Read the model definition and answer for the solid it produces. Units are mm, in the model's axes. A direction names the side the tool comes from. Round coordinates to 2 decimals unless told otherwise and drop trailing zeros. Write each loop counter-clockwise with the first axis right and the second up, starting at its lowest first coordinate (ties: lowest second). Pieces come first, ordered by that corner, then holes.
from build123d import *
from build123d.topology import SkipClean

# Parameters (mm, degrees)
SALIENTE_EXTRUIR1_DEPTH    = 2.4
CORTAR_EXTRUIR1_DEPTH      = 36.210225787
CORTAR_EXTRUIR1_DEPTH_BACK = 36.210225787
CROQUIS2_R                 = 1.5
CROQUIS3_R                 = 1.5
SALIENTE_EXTRUIR2_DEPTH    = 7.5
CORTAR_EXTRUIR2_DEPTH      = 3.1
REDONDEO1_R                = 2
REDONDEO2_R                = 1


with BuildPart() as part:
    # Croquis1 → Saliente-Extruir1 (new, symmetric)
    with BuildSketch(Plane(origin=(0, 0, 0), x_dir=(0, 0, -1), z_dir=(1, 0, 0))):
        with BuildLine():
            Line((-34, 3), (34, 3))
            ThreePointArc((34, 3), (34.707106781, 2.707106781), (35, 2))
            Line((35, 2), (35, -2))
            ThreePointArc((35, -2), (34.707106781, -2.707106781), (34, -3))
            Line((34, -3), (-34, -3))
            ThreePointArc((-34, -3), (-34.707106781, -2.707106781), (-35, -2))
            Line((-35, -2), (-35, 2))
            ThreePointArc((-35, 2), (-34.707106781, 2.707106781), (-34, 3))
        make_face()
    extrude(amount=SALIENTE_EXTRUIR1_DEPTH, both=True)

    # Croquis2 → Cortar-Extruir1 (cut, two sides: drawn at the far end of the back side and taken through both)
    with BuildSketch(Plane(origin=(0, 0, 0), x_dir=(0, 0, -1), z_dir=(1, 0, 0)).offset(-CORTAR_EXTRUIR1_DEPTH_BACK)):
        with Locations((-31, 0)):
            Circle(CROQUIS2_R)
        with Locations((31, 0)):
            Circle(CROQUIS2_R)
    extrude(amount=CORTAR_EXTRUIR1_DEPTH + CORTAR_EXTRUIR1_DEPTH_BACK, mode=Mode.SUBTRACT)

    # Croquis3 → Saliente-Extruir2 (add, symmetric)
    with SkipClean():  # the faces are left unmerged after this step: merging them gives an invalid solid
        with BuildSketch(Plane(origin=(0, 0, 0), x_dir=(0, 0, -1), z_dir=(1, 0, 0))):
            with BuildLine():
                Line((-35, 2), (-35, -2))
                ThreePointArc((-35, -2), (-34.707106781, -2.707106781), (-34, -3))
                Line((-34, -3), (-20, -3))
                Line((-20, -3), (-20, 3))
                Line((-20, 3), (-34, 3))
                ThreePointArc((-34, 3), (-34.707106781, 2.707106781), (-35, 2))
            make_face()
            with Locations((-31, 0)):
                Circle(CROQUIS3_R, mode=Mode.SUBTRACT)
        extrude(amount=SALIENTE_EXTRUIR2_DEPTH, both=True)
    add(part.part.scale(1), mode=Mode.REPLACE)  # the faces are merged on a copy

    # Croquis4 → Cortar-Extruir2 (cut, symmetric)
    with BuildSketch(Plane(origin=(0, 0, 0), x_dir=(0, 0, -1), z_dir=(1, 0, 0))):
        with BuildLine():
            Line((-34, 3), (-25, 3))
            Line((-25, 3), (-25, -3))
            Line((-25, -3), (-34, -3))
            ThreePointArc((-34, -3), (-34.707106781, -2.707106781), (-35, -2))
            Line((-35, -2), (-35, 2))
            ThreePointArc((-35, 2), (-34.707106781, 2.707106781), (-34, 3))
        make_face()
    extrude(amount=CORTAR_EXTRUIR2_DEPTH, both=True, mode=Mode.SUBTRACT)

    # Redondeo1
    redondeo1_edges = [part.edges().sort_by_distance(p)[0] for p in [
        (-2.4, 0, 20),
        (2.4, 0, 20),
        (-7.5, 0, 20),
        (7.5, 0, 20),
    ]]
    fillet(redondeo1_edges, radius=REDONDEO1_R)

    # Redondeo2
    redondeo2_edges = [part.edges().sort_by_distance(p)[0] for p in [
        (3.1, 0, 25),
        (-3.1, 0, 25),
    ]]
    fillet(redondeo2_edges, radius=REDONDEO2_R)


solid = part.part
Q1. Straight lines are drawn through the part: probe 1 along Y at (x, z) = (1.4, -31); probe 2 along X at (y, z) = (-1.75, 26); probe 3 along X at (y, z) = (2.25, 7). For each, find the intervals that lie inside material, in ascending order.
Verdict:
probe 1: y = -3 to -1.5, 1.5 to 3
probe 2: x = -7.5 to -3.1, 3.1 to 7.5
probe 3: x = -2.4 to 2.4
Q2. Flat-ended cylindrical pins translate along their axes: pin 1 Ø1.3 at (x, y) = (-1, 1) entering from +Z; pin 2 Ø2.5 at (y, z) = (0, 31) entering from +X; pin 3 Ø0.6 at (x, y) = (5, 1.5) entering from -Z; pin 4 Ø3 at (y, z) = (-2.5, 6.5) entering from -X. Find the tip coordinate at first contact, or state that the pin passes through.
Verdict:
pin 1: stops at z = 25
pin 2: passes through
pin 3: stops at z = 20
pin 4: stops at x = -2.4
Q3. Determine the mould class of faces 5 (the cylindrical face through (-5.3, -0.9, 32.2)), 6 (the cylindrical face through (6.9, 0.04, 20.57)), 7 (the flat face through (3.1, 0, 29)) for opening direction Z: pulls with the +Z half, pulls with the -Z half, needs draft (parallel to the pull), parting line crosses it, or undercut.
Verdict:
face 5: undercut
face 6: pulls with the -Z half
face 7: needs draft
Q4. Section B-B (y = 0.75) is taken. State how many separate pieces and enclosed holes the cut face has, then the cut area to 3 significant figures.
Verdict:
separate pieces: 4
enclosed holes: 0
area: 392 mm2
Q5. Which of the six approach directions +Z, -Z, +X, -X, +Y, -Y give full straight-line access (tool end or side, diameter ignored) to faces 1 (the flat face through (-3.1, 0, 29)), 2 (the flat face through (-2.4, 0, -9)), 3 (the flat face through (0, 3, 7)), 4 (the flat face through (5, 0, 20))?
Verdict:
face 1: +Z, +Y, -Y
face 2: -Z, -X, +Y, -Y
face 3: +Z, -Z, +X, -X, +Y
face 4: -Z, +X, +Y, -Y
Q6. Section D-D (z = 3.5) is taken. Determine the outline of the cut face in (x, y).
Verdict:
outline: (-2.4, -3) - (2.4, -3) - (2.4, 3) - (-2.4, 3) - close
Q7. Section C-C (x = 6.25) is taken. Determine the outline of the cut face in (y, z).
Verdict:
outline: (-3, 20.15) - (3, 20.15) - (3, 34) arc R1 ccw to (2, 35) - (-2, 35) arc R1 ccw to (-3, 34) - close; hole circle Ø3 at (0, 31)
Q8. Section A-A (z = 31) is taken. Determine the outline of the cut face in (x, y), then the cut area to 3 significant figures.
Verdict:
outline: (-7.5, -3) - (-3.1, -3) - (-3.1, -1.5) - (-7.5, -1.5) - close; (-7.5, 1.5) - (-3.1, 1.5) - (-3.1, 3) - (-7.5, 3) - close; (3.1, -3) - (7.5, -3) - (7.5, -1.5) - (3.1, -1.5) - close; (3.1, 1.5) - (7.5, 1.5) - (7.5, 3) - (3.1, 3) - close
area: 26.4 mm2
